Geometry: final body of the model. Coordinates: model frame, mm. A direction names the side the tool comes from. Give positions to 0.01 mm unless a question says otherwise; leave off trailing zeros. Write each loop counter-clockwise with the first axis right and the second up, starting at its lowest first coordinate (ties: lowest second). Pieces come first, ordered by that corner, then holes. Notation, with made-up numbers: (-34.75, 29) -> (-1.75, 29) arc R15 cw to (-1.75, 46) -> close; hole circle Ø8 at (31, 53.25). An arc over 180 degrees is marked (long way). Answer as a JSON object with one key per item and string values. Group by question number.
(1) Set-up query: faces 4 (the face through (183.57, 64.993, 33.24)), 5 (the face through (32.317, 71.944, 52.407)). Return all of +Z, -Z, +X, -X, +Y, -Y with unobstructed straight access to the full face (end or side cutting, diameter ignored); none if empty.
(2) Section query D-D on x = 23. Output: boundary loops of the cut face in (y, z), plus the area to 3 significant figures.
(3) Section query C-C on z = 46.5. Output: boundary loops of the cut face in (x, y), plus the area to 3 significant figures.
(4) Contact query for flat-ended pins moving along their axis: pin 1 Ø0.8 at (x, z) = (69, 66) entering from +Y; pin 2 Ø1.1 at (y, z) = (1.5, 66) entering from -X; pin 3 Ø1.1 at (y, z) = (1.5, 66.5) entering from +X. Output: stop coordinate, or through.
(5) Draft query along Y for faces 1 (the face through (24, 0, 34)), 2 (the face through (-130.73, 64.99, 33.24)), 3 (the face through (26, 9, 65.688)). Return one class per face: +Y half, -Y half, draft (parallel to the pull), parting line (faces both ways), or undercut.
(6) Section query B-B on z = 60. Output: boundary loops of the cut face in (x, y).
(7) Material intervals for probe 1 along Y at (x, z) = (58, 47); probe 2 along X at (y, z) = (59, 33.5); probe 3 along Z at (x, y) = (90, 5), sorted ascending.
(8) Section query A-A on x = 137.5. Output: boundary loops of the cut face in (y, z).
from build123d import *

# Parameters (mm, degrees)
SKETCH_1_W      = 320
SKETCH_1_H      = 64
EXTRUDE_1_DEPTH = 68
FILLET_1_R      = 10
SKETCH_2_R      = 19.624889804
EXTRUDE_2_DEPTH = 8
SKETCH_3_W      = 300
SKETCH_3_H      = 50.287952294
SKETCH_3_H_2    = 4.344723496
EXTRUDE_3_DEPTH = 1


with BuildPart() as part:
    # 草图1 → 凸台-拉伸1 (new body)
    with BuildSketch(Plane(origin=(0, 0, 0), x_dir=(1, 0, 0), z_dir=(0, 1, 0))):
        with Locations((26.422018349, -33.688073394)):
            Rectangle(SKETCH_1_W, SKETCH_1_H)
    extrude(amount=EXTRUDE_1_DEPTH)

    # 圆角1
    fillet_1_edges = [part.edges().sort_by_distance(p)[0] for p in [
        (186.422018349, 68, 33.688073394),
        (-133.577981651, 68, 33.688073394),
        (186.422018349, 0, 33.688073394),
        (-133.577981651, 0, 33.688073394),
    ]]
    fillet(fillet_1_edges, radius=FILLET_1_R)

    # 草图2 → 凸台-拉伸2 (add)
    with BuildSketch(Plane(origin=(0, 68, 0), x_dir=(1, 0, 0), z_dir=(0, 1, 0))):
        with Locations(Location((26.422018349, -33.688073394, 0), (0, 0, 270))):
            Circle(SKETCH_2_R)
    extrude(amount=EXTRUDE_2_DEPTH)

    # 草图3 → 凸台-拉伸3 (add)
    with BuildSketch(Plane.XY.offset(65.688073394)):
        with Locations((26.422018349, 36.856023853)):
            Rectangle(SKETCH_3_W, SKETCH_3_H)
        with Locations((26.422018349, 2.172361748)):
            Rectangle(SKETCH_3_W, SKETCH_3_H_2)
    extrude(amount=EXTRUDE_3_DEPTH)


solid = part.part
Answer list:
{
 "1": {"face 4": "+Z, -Z, +X, +Y", "face 5": "+Y"},
 "2": {"outline": "(0, 1.69) -> (68, 1.69) -> (68, 14.36) -> (76, 14.36) -> (76, 53.01) -> (68, 53.01) -> (68, 65.69) -> (62, 65.69) -> (62, 66.69) -> (11.71, 66.69) -> (11.71, 65.69) -> (4.34, 65.69) -> (4.34, 66.69) -> (0, 66.69) -> close", "area": "4,720 mm2"},
 "3": {"outline": "(-133.58, 10) arc R10 ccw to (-123.58, 0) -> (176.42, 0) arc R10 ccw to (186.42, 10) -> (186.42, 58) arc R10 ccw to (176.42, 68) -> (41.29, 68) -> (41.29, 76) -> (11.56, 76) -> (11.56, 68) -> (-123.58, 68) arc R10 ccw to (-133.58, 58) -> close", "area": "21,900 mm2"},
 "4": {"pin 1": "y = 68", "pin 2": "x = -129.51", "pin 3": "x = 176.42"},
 "5": {"face 1": "-Y half", "face 2": "+Y half", "face 3": "undercut"},
 "6": {"outline": "(-133.58, 10) arc R10 ccw to (-123.58, 0) -> (176.42, 0) arc R10 ccw to (186.42, 10) -> (186.42, 58) arc R10 ccw to (176.42, 68) -> (-123.58, 68) arc R10 ccw to (-133.58, 58) -> close"},
 "7": {"probe 1": "0 to 68", "probe 2": "-133.53 to 186.37", "probe 3": "1.69 to 65.69"},
 "8": {"outline": "(0, 1.69) -> (68, 1.69) -> (68, 65.69) -> (62, 65.69) -> (62, 66.69) -> (11.71, 66.69) -> (11.71, 65.69) -> (4.34, 65.69) -> (4.34, 66.69) -> (0, 66.69) -> close"}
}
